Geometry: see drawing. Coordinates: mm, zero at the bounding-box minimum. Give positions to 0.01 mm unless a question says otherwise; leave off trailing zeros. Loops run counter-clockwise (first coordinate to the right, second up) from the corner with the lowest first, then second, coordinate; pieces in that order, holes last. Notation, with made-up numbers: (-36.75, 60.25) - (20.25, 60.25) arc R10 ccw to (20.25, 71.25) - close; hole circle Ø10 at (-19, 47). An arc over 180 degrees is marked (long way). Use one line per item in the form item = value.
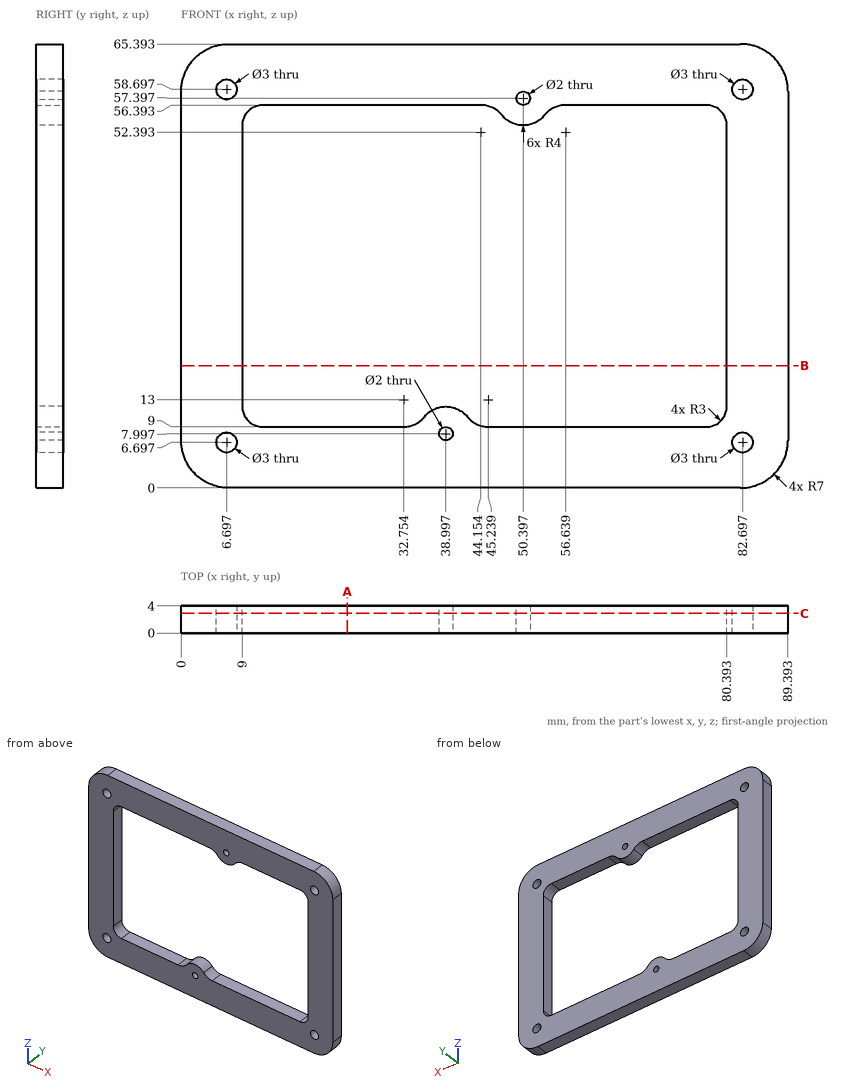
(1) Cut plane C-C (y = 2.9). Give the number of separate pieces and of enclosed holes in the cut face, plus the area to 3 significant figures.
Solution:
separate_pieces = 1
enclosed_holes = 7
area = 2,430 mm2
(2) Material intervals for L1, parallel to Z at x = 18.5, y = 2.7; L2, parallel to X at y = 1.75, z = 29.5; L3, parallel to X at y = 1.95, z = 11 (1 decimal), sorted ascending. Write a range as from..to.
Solution:
L1 = 0..9, 56.39..65.39
L2 = 0..9, 80.39..89.39
L3 = 0..9.2, 36.4..41.6, 80.2..89.4
(3) Pin query (flat end, axial travel): P1, Ø2.5, axis at x = 82.7, z = 58.7, coming from the -Y side. Return the tip coordinate at first contact, or that it passes through.
Solution:
P1 = through
(4) Cut plane B-B (z = 18). Return the cut outline in (x, y), plus the area to 3 significant figures.
Solution:
outline = (0, 0) - (9, 0) - (9, 4) - (0, 4) - close; (80.39, 0) - (89.39, 0) - (89.39, 4) - (80.39, 4) - close
area = 72.0 mm2
(5) Cut plane A-A (x = 24.5). Return the cut outline in (y, z), plus the area to 3 significant figures.
Solution:
outline = (0, 0) - (4, 0) - (4, 9) - (0, 9) - close; (0, 56.39) - (4, 56.39) - (4, 65.39) - (0, 65.39) - close
area = 72.0 mm2
